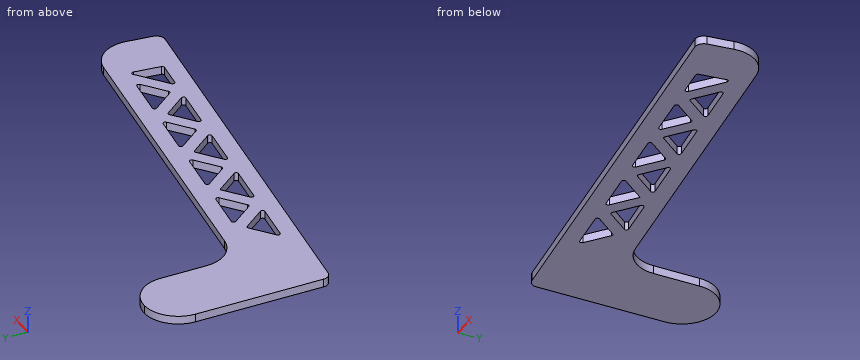
from build123d import *

# Parameters (mm, degrees)
SKETCH1_R           = 7.9375
SKETCH1_R_2         = 4.7879
BOSS_EXTRUDE1_DEPTH = 4.7625
FILLET3_R           = 40
FILLET4_R           = 10
CUT_EXTRUDE1_DEPTH  = 10
FILLET5_R           = 2.5
SKETCH30_R          = 7.9375
SKETCH30_R_2        = 4.7879
BOSS_EXTRUDE2_DEPTH = 9.525


with BuildPart() as part:
    # Sketch1 → Boss-Extrude1 (new, symmetric)
    with BuildSketch(Plane.XY):
        Polygon((-144.07836487, 49.742763384), (-144.07836487, -50.257236616), (365.353249064, -113.421723532), (375.197079951, -34.029664776), (-64.07836487, 20.436150317), (-64.07836487, 149.742763384), (-144.07836487, 149.742763384), align=None)
        with Locations(Location((-104.07836487, 109.742763384, 0), (0, 0, 180))):
            Circle(SKETCH1_R, mode=Mode.SUBTRACT)
        with Locations(Location((330.57913513, -68.80377871, 0), (0, 0, 180))):
            Circle(SKETCH1_R_2, mode=Mode.SUBTRACT)
    extrude(amount=BOSS_EXTRUDE1_DEPTH, both=True)

    # Fillet3
    fillet3_edges = [part.edges().sort_by_distance(p)[0] for p in [
        (-64.07836487, 20.436150317, 0),
        (-64.07836487, 149.742763384, 0),
        (-144.07836487, 149.742763384, 0),
        (375.197079951, -34.029664776, 0),
    ]]
    fillet(fillet3_edges, radius=FILLET3_R - 0.0001)  # a hair under: the kernel refuses the full size

    # Fillet4
    fillet4_edges = [part.edges().sort_by_distance(p)[0] for p in [
        (365.353249064, -113.421723532, 0),
        (-144.07836487, -50.257236616, 0),
    ]]
    fillet(fillet4_edges, radius=FILLET4_R)

    # Sketch16 → Cut-Extrude1 (cut)
    with BuildSketch(Plane.XY.offset(4.7625)):
        Polygon((54.565895217, -14.427714854), (-3.774164869, -7.194123807), (21.77906965, -39.980949374), align=None)
        Polygon((-15.605284124, -16.415003221), (-48.392109691, -41.968237741), (9.947950395, -49.201828788), align=None)
        Polygon((133.957953972, -24.271545742), (75.617893886, -17.037954695), (101.171128405, -49.824780261), align=None)
        Polygon((63.786774631, -26.258834109), (30.999949065, -51.812068628), (89.340009151, -59.045659676), align=None)
        Polygon((213.350012728, -34.11537663), (155.009952642, -26.881785582), (180.563187161, -59.668611149), align=None)
        Polygon((143.178833387, -36.102664997), (110.39200782, -61.655899516), (168.732067906, -68.889490564), align=None)
        Polygon((292.742071484, -43.959207518), (234.402011397, -36.72561647), (259.955245917, -69.512442037), align=None)
        Polygon((222.570892143, -45.946495885), (189.784066576, -71.499730404), (248.124126662, -78.733321452), align=None)
        Polygon((313.794070153, -46.569447358), (269.176125331, -81.343561292), (308.872154709, -86.265476736), align=None)
    extrude(amount=-CUT_EXTRUDE1_DEPTH, mode=Mode.SUBTRACT)

    # Fillet5
    fillet5_edges = [part.edges().sort_by_distance(p)[0] for p in [
        (110.39200782, -61.655899516, 0),
        (143.178833387, -36.102664997, 0),
        (168.732067906, -68.889490564, 0),
        (292.742071484, -43.959207518, 0),
        (259.955245917, -69.512442037, 0),
        (234.402011397, -36.72561647, 0),
        (189.784066576, -71.499730404, 0),
        (222.570892143, -45.946495885, 0),
        (248.124126662, -78.733321452, 0),
        (-48.392109691, -41.968237741, 0),
        (-15.605284124, -16.415003221, 0),
        (9.947950395, -49.201828788, 0),
        (30.999949065, -51.812068628, 0),
        (89.340009151, -59.045659676, 0),
        (54.565895217, -14.427714854, 0),
        (21.77906965, -39.980949374, 0),
        (-3.774164869, -7.194123807, 0),
        (133.957953972, -24.271545742, 0),
        (101.171128405, -49.824780261, 0),
        (75.617893886, -17.037954695, 0),
        (269.176125331, -81.343561292, 0),
        (313.794070153, -46.569447358, 0),
        (308.872154709, -86.265476736, 0),
        (213.350012728, -34.11537663, 0),
        (180.563187161, -59.668611149, 0),
        (155.009952642, -26.881785582, 0),
    ]]
    fillet(fillet5_edges, radius=FILLET5_R)

    # Sketch30 → Boss-Extrude2 (add)
    with BuildSketch(Plane(origin=(0, 0, -4.7625), x_dir=(-1, 0, 0), z_dir=(0, 0, -1))):
        with Locations((104.07836487, 109.742763384)):
            Circle(SKETCH30_R)
        with Locations((-330.57913513, -68.80377871)):
            Circle(SKETCH30_R_2)
    extrude(amount=-BOSS_EXTRUDE2_DEPTH)


solid = part.part
Geometry check sheet. Reference: the model listing, model coordinates, mm. Round coordinates to 2 decimals unless told otherwise and drop trailing zeros. Order: outer loops, then holes, each group sorted by start corner. A loop starts at its lowest first (then second) coordinate and runs counter-clockwise, first axis right, second up. Notation, with made-up numbers: (-33, 7.5) -> (1, 7.5) arc R24 cw to (1, 28.5) -> close; hole circle Ø8 at (3, 65). An arc over 180 degrees is marked (long way). Use one line per item in the form item = value.
1. Scan lines: line 1 along Y through (x, z) = (284.5, -0.5); line 2 along Y through (x, z) = (114.5, 3.5); line 3 along X through (y, z) = (111, 0.25). Record each from-to range of solid material in increasing order. Write a range as from..to.
Working result:
line_1 = -103.4..-83.24, -69.4..-50.38, -42.94..-22.78
line_2 = -82.32..-61.12, -58.71..-39.44, -21.86..-1.71
line_3 = -144.06..-64.1
2. Cross-section at B-B, the plane y = -96. Enter the section's corners in (x, z).
Working result:
outline = (224.84, -4.76) -> (367.51, -4.76) -> (367.51, 4.76) -> (224.84, 4.76) -> close
3. Go/stop test with flat-tipped pins: pin 1 (1 mm diameter, centred on x = 67.5, z = 0.5, fed in from -Y); pin 2 (4 mm diameter, centred on x = -89, z = -2.5, fed in from +Y); pin 3 (5 mm diameter, centred on y = 52.5, z = 2.5, fed in from +X). Record where each tip stops, or that it passes through.
Working result:
pin_1 = -76.55
pin_2 = 147.54
pin_3 = -63.66
4. Cross-section at C-C, the plane x = -84. Enter the section's corners in (y, z), plus the area to 3 significant figures.
Working result:
outline = (-57.71, -4.76) -> (144.34, -4.76) -> (144.34, 4.76) -> (-57.71, 4.76) -> close
area = 1,920 mm^2
5. Cross-section at A-A, the plane z = -0.75. Count the separate pieces of the cut face and the enclosed holes in it, plus the area to 3 significant figures.
Working result:
separate_pieces = 1
enclosed_holes = 9
area = 43,000 mm^2
